```python
from build123d import *

# Parameters (mm, degrees)
F1_DEPTH = 5
F2_DEPTH = 5
F0_R     = 1.25
F3_DEPTH = 2.5


with BuildPart() as f1:
    # F0 (on Front) → F1 (new body, symmetric)
    with BuildSketch(Plane.XZ):
        with BuildLine():
            Line((-9, 0), (-9, 44))
            Line((-9, 44), (0, 44))
            Line((0, 44), (0, 49))
            add(Edge.make_bspline(
                [(-19.43566, 63.521571), (-13.189036, 59.186175), (-6.594518, 49), (0, 49)],
                knots=[0, 0, 0, 0, 24.261511, 24.261511, 24.261511, 24.261511], degree=3))
            ThreePointArc((-19.43566, 63.521571), (-19.43566, 52.256946), (-30.700285, 52.256946))
            add(Edge.make_bspline(
                [(-14, 0), (-14, 17.46672), (-23.267117, 34.933441), (-30.700285, 52.256946)],
                knots=[54.860623, 54.860623, 54.860623, 54.860623, 109.721246, 109.721246, 109.721246, 109.721246], degree=3))
            Line((-14, 0), (-9, 0))
        make_face()
        with BuildLine():
            Line((0, 49), (0, 44))
            Line((0, 44), (9, 44))
            Line((9, 44), (9, -44))
            Line((9, -44), (-9, -44))
            Line((-9, -44), (-9, 0))
            Line((-9, 0), (-14, 0))
            add(Edge.make_bspline(
                [(-30.700285, -52.256946), (-23.267117, -34.933441), (-14, -17.46672), (-14, 0)],
                knots=[0, 0, 0, 0, 54.860623, 54.860623, 54.860623, 54.860623], degree=3))
            ThreePointArc((-30.700285, -52.256946), (-24.914376, -49.925447), (-19.222671, -52.478313))
            ThreePointArc((-19.222671, -52.478313), (-17.104161, -58.042855), (-19.43566, -63.521571))
            add(Edge.make_bspline(
                [(-19.43566, -63.521571), (-13.189036, -59.186175), (0, -38.813825), (13.189036, -59.186175), (19.43566, -63.521571)],
                knots=[0, 0, 0, 0, 24.261511, 48.523022, 48.523022, 48.523022, 48.523022], degree=3))
            ThreePointArc((19.43566, -63.521571), (19.43566, -52.256946), (30.700285, -52.256946))
            add(Edge.make_bspline(
                [(30.700285, -52.256946), (23.267117, -34.933441), (4.732883, 0), (23.267117, 34.933441), (30.700285, 52.256946)],
                knots=[0, 0, 0, 0, 54.860623, 109.721246, 109.721246, 109.721246, 109.721246], degree=3))
            ThreePointArc((30.700285, 52.256946), (19.43566, 52.256946), (19.43566, 63.521571))
            add(Edge.make_bspline(
                [(0, 49), (6.594518, 49), (13.189036, 59.186175), (19.43566, 63.521571)],
                knots=[24.261511, 24.261511, 24.261511, 24.261511, 48.523022, 48.523022, 48.523022, 48.523022], degree=3))
        make_face()
    extrude(amount=F1_DEPTH, both=True)

    # F0 (on Front) → F2 (join)
    with BuildSketch(Plane.XZ):
        Polygon((0, 44), (-9, 44), (-9, 0), (-9, -44), (9, -44), (9, 44), align=None)
    extrude(amount=-F2_DEPTH)

    # F0 (on Front) → F3 (join, symmetric)
    with BuildSketch(Plane.XZ):
        with BuildLine():
            ThreePointArc((-30.700285, 52.256946), (-19.43566, 52.256946), (-19.43566, 63.521571))
            Line((-19.43566, 63.521571), (-26.604424, 70.690334))
            ThreePointArc((-26.604424, 70.690334), (-34.333678, 67.072101), (-37.480628, 59.139279))
            Line((-37.480628, 59.139279), (-30.700285, 52.256946))
        make_face()
        with Locations((-29.82286, 63.078503)):
            Circle(F0_R, mode=Mode.SUBTRACT)
        with Locations((-25.908636, 54.921638)):
            Circle(F0_R, mode=Mode.SUBTRACT)
        with Locations((-21.908602, 59.186175)):
            Circle(F0_R, mode=Mode.SUBTRACT)
        with BuildLine():
            Line((26.604424, 70.690334), (19.43566, 63.521571))
            ThreePointArc((19.43566, 63.521571), (19.43566, 52.256946), (30.700285, 52.256946))
            Line((30.700285, 52.256946), (37.480628, 59.139279))
            ThreePointArc((37.480628, 59.139279), (34.333678, 67.072101), (26.604424, 70.690334))
        make_face()
        with Locations((21.908602, 59.186175)):
            Circle(F0_R, mode=Mode.SUBTRACT)
        with Locations((25.908636, 54.921638)):
            Circle(F0_R, mode=Mode.SUBTRACT)
        with Locations((29.82286, 63.078503)):
            Circle(F0_R, mode=Mode.SUBTRACT)
        with BuildLine():
            Line((37.480628, -59.139279), (30.700285, -52.256946))
            ThreePointArc((30.700285, -52.256946), (19.43566, -52.256946), (19.43566, -63.521571))
            Line((19.43566, -63.521571), (26.604424, -70.690334))
            ThreePointArc((26.604424, -70.690334), (34.333678, -67.072101), (37.480628, -59.139279))
        make_face()
        with Locations((21.908602, -59.186175)):
            Circle(F0_R, mode=Mode.SUBTRACT)
        with Locations((25.908636, -54.921638)):
            Circle(F0_R, mode=Mode.SUBTRACT)
        with Locations((29.82286, -63.078503)):
            Circle(F0_R, mode=Mode.SUBTRACT)
        with BuildLine():
            ThreePointArc((-19.222671, -52.478313), (-24.914376, -49.925447), (-30.700285, -52.256946))
            Line((-30.700285, -52.256946), (-37.480628, -59.139279))
            ThreePointArc((-37.480628, -59.139279), (-34.333678, -67.072101), (-26.604424, -70.690334))
            Line((-26.604424, -70.690334), (-19.43566, -63.521571))
            ThreePointArc((-19.43566, -63.521571), (-17.104161, -58.042855), (-19.222671, -52.478313))
        make_face()
        with BuildLine():
            ThreePointArc((-28.57286, -63.078503), (-30.977709, -63.556857), (-28.938977, -62.194619))
            ThreePointArc((-28.938977, -62.194619), (-28.668011, -62.600148), (-28.57286, -63.078503))
        make_face(mode=Mode.SUBTRACT)
        with Locations((-25.908636, -54.921638)):
            Circle(F0_R, mode=Mode.SUBTRACT)
        with Locations((-21.908602, -59.186175)):
            Circle(F0_R, mode=Mode.SUBTRACT)
    extrude(amount=F3_DEPTH, both=True)


solid = f1.part
```
CAD build for the part. Positions are in the model's coordinates, mm. A direction names the side the tool comes from. Coordinates: 2 decimals unless noted, no trailing zeros. Order: outer loops, then holes, each group sorted by start corner. A loop starts at its lowest first (then second) coordinate and runs counter-clockwise, first axis right, second up. Notation, with made-up numbers: M -34,70 L -30,70 A22 cw -30,80 Z; hole C 2.5,-2 d10. An arc over 180 degrees is marked long. Write each question's results on one line, items separated by ' | '. Start each with the question number.
Q1. Pull direction X, two halves, no side cores. Call faces 1 (the flat face through (0, 5, 1)), 2 (the flat face through (0, -3, 44)), 3 (the flat face through (-34.043, -0.035, -55.65)): +X half, -X half, draft (parallel to the pull), parting line (faces both ways), or undercut.
Q2. Which spindle directions (+Z, -Z, +X, -X, +Y, -Y) get a long thin tool onto all of the face, cutting with end or side? Do faces 4 (the flat face through (9, -3, 1)), 5 (the cylindrical face through (-19.313, 3.732, 52.382)), 6 (the flat face through (-22.97, 0.035, 67.056)). Say none if no direction does.
Q3. Cut at A-A (x = 33). List the corners of the cut face in (y, z), then the cut area to 3 significant figures.
Q4. Flat gauge pins, fed straight in: P1, Ø3, axis at y = -0.5, z = 17.5, coming from the -X side; P2, Ø3, axis at x = 29.82, z = 63.08, coming from the +Y side; P3, Ø3, axis at y = -1.5, z = 42, coming from the +X side; P4, Ø2, axis at x = 29.82, z = -63.08, coming from the -Y side. Where does each tip first touch, or does it go through?
Q5. Drill centre lines: probe 1 along Z at (x, y) = (30, 2.25); probe 2 along Z at (x, y) = (-23, 1.5); probe 3 along Z at (x, y) = (-27.5, -3.5). Where is each one in solid material? Low to high. Write a range as from..to.
Found:
1) face 1: draft | face 2: undercut | face 3: -X half
2) face 4: -Y | face 5: +Y | face 6: +Z, +Y, -Y
3) outline: M -2.5,-68.28 L 2.5,-68.28 L 2.5,-54.59 L -2.5,-54.59 Z; M -2.5,54.59 L 2.5,54.59 L 2.5,68.28 L -2.5,68.28 Z | area: 137 mm²
4) P1: x = -17.13 | P2: y = 2.5 | P3: x = 26.84 | P4: through
5) probe 1: -69.96..-64.32, -61.84..-50.64, 50.64..61.84, 64.32..69.96 | probe 2: -67.09..-59.8, -58.58..-34.73, 34.73..58.58, 59.8..67.09 | probe 3: -50.3..-44.97, 44.97..50.3
